The model under review builds one solid part; all positions refer to its coordinate system, in mm. Face numbers are marked on the shaded views. A direction names the side the tool comes from. Give positions to 0.01 mm unless a question says otherwise; leave off trailing zeros. Write each loop counter-clockwise with the first axis right and the second up, starting at its lowest first coordinate (ties: lowest second). Pieces come first, ordered by that corner, then holes. Notation, with made-up numbers: (72.25, -3) - (92.25, -3) arc R15 cw to (92.25, 24) - close; hole circle Ø11 at (41, 24). An arc over 180 degrees is marked (long way). Write item = value, one per line.
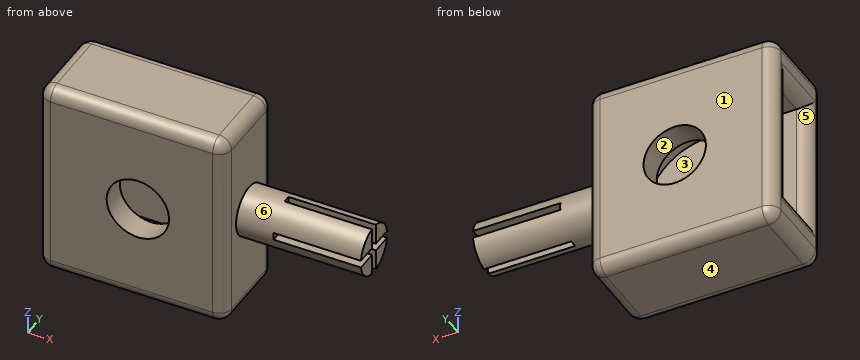
```python
from build123d import *

# Parameters (mm, degrees)
BOSS_EXTRUDE1_DEPTH = 3.2
SKETCH2_W           = 15
SKETCH2_H           = 16.1
BOSS_EXTRUDE2_DEPTH = 2
SKETCH3_W           = 15
SKETCH3_H           = 16.1
BOSS_EXTRUDE3_DEPTH = 2
FILLET1_R           = 1
SKETCH4_R           = 2
BOSS_EXTRUDE4_DEPTH = 10
CUT_EXTRUDE1_START  = -7
CUT_EXTRUDE1_DEPTH  = 7
SKETCH6_R           = 2.5
CUT_EXTRUDE2_DEPTH  = 31.594934221


with BuildPart() as part:
    # Sketch1 → Boss-Extrude1 (new body)
    with BuildSketch(Plane(origin=(0, 0, 0), x_dir=(1, 0, 0), z_dir=(0, 1, 0))):
        with BuildLine():
            Line((0, 13.1), (0, 16.1))
            Line((0, 16.1), (15, 16.1))
            Line((15, 16.1), (15, 0))
            Line((15, 0), (0, 0))
            Line((0, 0), (0, 3))
            Line((0, 3), (8, 3))
            ThreePointArc((8, 3), (13.05, 8.05), (8, 13.1))
            Line((8, 13.1), (0, 13.1))
        make_face()
    extrude(amount=BOSS_EXTRUDE1_DEPTH)

    # Sketch2 → Boss-Extrude2 (add)
    with BuildSketch(Plane(origin=(0, 3.2, 0), x_dir=(1, 0, 0), z_dir=(0, 1, 0))):
        with Locations((7.5, 8.05)):
            Rectangle(SKETCH2_W, SKETCH2_H)
    extrude(amount=BOSS_EXTRUDE2_DEPTH)

    # Sketch3 → Boss-Extrude3 (add)
    with BuildSketch(Plane.XZ):
        with Locations((7.5, -8.05)):
            Rectangle(SKETCH3_W, SKETCH3_H)
    extrude(amount=BOSS_EXTRUDE3_DEPTH)

    # Fillet1
    fillet1_edges = [part.edges().sort_by_distance(p)[0] for p in [
        (0, 1.6, -3),
        (0, 1.6, -13.1),
        (0, 1.6, -16.1),
        (15, 1.6, -16.1),
        (15, 1.6, 0),
        (0, 1.6, 0),
        (0, 3.2, -8.05),
        (15, 5.2, -8.05),
        (7.5, 5.2, -16.1),
        (0, 5.2, -8.05),
        (7.5, 5.2, 0),
        (0, 0, -8.05),
        (0, -2, -8.05),
        (7.5, -2, -16.1),
        (15, -2, -8.05),
        (7.5, -2, 0),
    ]]
    fillet(fillet1_edges, radius=FILLET1_R - 0.0001)  # a hair under: the kernel refuses the full size

    # Sketch4 → Boss-Extrude4 (add)
    with BuildSketch(Plane(origin=(15, 0, 0), x_dir=(0, 0, -1), z_dir=(1, 0, 0))):
        with Locations(Location((8.05, 1.65, 0), (0, 0, 180))):
            Circle(SKETCH4_R)
    extrude(amount=BOSS_EXTRUDE4_DEPTH)

    # Sketch5 → Cut-Extrude1 (cut)
    with BuildSketch(Plane(origin=(25, 0, 0), x_dir=(0, 0, -1), z_dir=(1, 0, 0)).offset(CUT_EXTRUDE1_START)):
        with BuildLine():
            Line((6.072628007, 1.95), (7.75, 1.95))
            Line((7.75, 1.95), (7.75, 3.627371993))
            ThreePointArc((7.75, 3.627371993), (8.05, 3.65), (8.35, 3.627371993))
            Line((8.35, 3.627371993), (8.35, 1.95))
            Line((8.35, 1.95), (10.027371993, 1.95))
            ThreePointArc((10.027371993, 1.95), (10.05, 1.65), (10.027371993, 1.35))
            Line((10.027371993, 1.35), (8.35, 1.35))
            Line((8.35, 1.35), (8.35, -0.327371993))
            ThreePointArc((8.35, -0.327371993), (8.05, -0.35), (7.75, -0.327371993))
            Line((7.75, -0.327371993), (7.75, 1.35))
            Line((7.75, 1.35), (6.072628007, 1.35))
            ThreePointArc((6.072628007, 1.35), (6.05, 1.65), (6.072628007, 1.95))
        make_face()
    extrude(amount=CUT_EXTRUDE1_DEPTH, mode=Mode.SUBTRACT)

    # Sketch6 → Cut-Extrude2 (cut, through all)
    with BuildSketch(Plane(origin=(0, 5.2, 0), x_dir=(1, 0, 0), z_dir=(0, 1, 0))):
        with Locations(Location((8, 8.05, 0), (0, 0, 270))):
            Circle(SKETCH6_R)
    extrude(amount=-CUT_EXTRUDE2_DEPTH, mode=Mode.SUBTRACT)


solid = part.part
```
1. Draft analysis for pull direction Y (two halves, no side actions). For the marked faces 1, 2 and 3, state which applies: +Y half, -Y half, draft (parallel to the pull), parting line (faces both ways), or undercut.
Findings below:
face_1 = +Y half
face_2 = draft
face_3 = undercut
2. Take a section at C-C on x = 1.75. Give the boundary of the cut face in (y, z).
Findings below:
outline = (-2, -15.1) arc R1 ccw to (-1, -16.1) - (4.2, -16.1) arc R1 ccw to (5.2, -15.1) - (5.2, -1) arc R1 ccw to (4.2, 0) - (-1, 0) arc R1 ccw to (-2, -1) - close; hole (0, -13.1) - (3.2, -13.1) - (3.2, -3) - (0, -3) - close
3. For line 1 (Y direction, x = 9.5, z = -5); line 2 (X direction, y = 4.1, z = -8.05) (3 decimals); line 3 (Z direction, x = 10, y = 0.5), list the stretches that pass through material, from the lowest coordinate up. Write a range as from..to.
Findings below:
line_1 = -2..0, 3.2..5.2
line_2 = 0.005..5.5, 10.5..15
line_3 = -16.1..-12.69, -3.41..0
4. Take a section at D-D on y = 4.5. Give the boundary of the cut face in (x, z).
Findings below:
outline = (0.05, -15.1) arc R0.95 ccw to (1, -16.05) - (14, -16.05) arc R0.95 ccw to (14.95, -15.1) - (14.95, -1) arc R0.95 ccw to (14, -0.05) - (1, -0.05) arc R0.95 ccw to (0.05, -1) - close; hole circle Ø5 at (8, -8.05)
5. Take a section at B-B on x = 20. Give the boundary of the cut face in (y, z), and give its area (3 significant figures).
Findings below:
outline = (-0.33, -8.35) arc R2 ccw to (1.35, -10.03) - (1.35, -8.35) - close; (-0.33, -7.75) - (1.35, -7.75) - (1.35, -6.07) arc R2 ccw to start; (1.95, -10.03) arc R2 ccw to (3.63, -8.35) - (1.95, -8.35) - close; (1.95, -7.75) - (3.63, -7.75) arc R2 ccw to (1.95, -6.07) - close
area = 8.14 mm²
6. Insertion check: P1, Ø0.5, axis at x = 21.5, y = 0, coming from the -Z side; P2, Ø0.5, axis at x = 21, y = 3, coming from the -Z side; P3, Ø1.5, axis at y = 3.5, z = -2.5, coming from the +X side; P4, Ø4.5, axis at x = 8, z = -8.05, coming from the -Y side. Each pin has a flat end and moves straight along its axis. Give the tip position at first contact, or say it passes through.
Findings below:
P1 = -9.48
P2 = -9.72
P3 = 15
P4 = through
7. Machinability: for the marked faces 4, 5 and 6, which of the approach directions +Z, -Z, +X, -X, +Y, -Y give a long, thin tool a straight path to every point of the face, cutting with its end or side? Answer none if there is none.
Findings below:
face_4 = -Z, +X, -X, +Y, -Y
face_5 = -X
face_6 = +X
8. Take a section at A-A on z = -8.05. Count the separate pieces of the cut face and the enclosed holes in it, and give its area (3 significant figures).
Findings below:
separate_pieces = 3
enclosed_holes = 0
area = 57.0 mm²
